Geometry check sheet. Reference: the model listing, model coordinates, mm. Face numbers are marked on the shaded views. A direction names the side the tool comes from. Coordinates: 2 decimals unless noted, no trailing zeros. Order: outer loops, then holes, each group sorted by start corner. A loop starts at its lowest first (then second) coordinate and runs counter-clockwise, first axis right, second up. Notation, with made-up numbers: (13.5, -12.5) -> (26.5, -12.5) arc R14 cw to (26.5, 1.5) -> close; hole circle Ø6 at (29, 72.5). An arc over 180 degrees is marked (long way). Answer in a Markdown table with one row per item. Add a question column.
```python
from build123d import *

# Parameters (mm, degrees)
EXTRUDE_1_DEPTH     = 100
FILLET_1_R          = 4
EXTRUDE_2_DEPTH     = 50
FILLET_2_R          = 1
CUT_EXTRUDE_1_DEPTH = 155.597772267
FILLET_3_R          = 1
CUT_EXTRUDE_2_REACH = 157.823
SKETCH_4_R          = 2.099999206


with BuildPart() as part:
    # 草图1 → 凸台-拉伸1 (new, symmetric)
    with BuildSketch(Plane.XY):
        Polygon((-30.1, 0), (30.1, 0), (0, 30.003999733), align=None)
    extrude(amount=EXTRUDE_1_DEPTH, both=True)

    # 圆角1
    fillet_1_edges = [part.edges().sort_by_distance(p)[0] for p in [
        (0, 30.003999733, 0),
        (30.1, 0, 0),
        (-30.1, 0, 0),
    ]]
    fillet(fillet_1_edges, radius=FILLET_1_R)

    # 草图2 → 凸台-拉伸2 (add)
    with BuildSketch(Plane.XY.offset(100)):
        Polygon((15.581935613, 6), (0, 21.532238936), (-15.581935613, 6), align=None)
    extrude(amount=EXTRUDE_2_DEPTH)

    # 圆角2
    fillet_2_edges = [part.edges().sort_by_distance(p)[0] for p in [
        (-15.581935613, 6, 125),
        (15.581935613, 6, 125),
        (0, 21.532238936, 125),
    ]]
    fillet(fillet_2_edges, radius=FILLET_2_R)

    # 草图3 → 切除-拉伸1 (cut, through all)
    with BuildSketch(Plane(origin=(0, 0, 0), x_dir=(1, 0, 0), z_dir=(0, 1, 0))):
        Polygon((-15, 82), (0, 67), (15, 82), align=None)
        Polygon((-8, 55), (-18, 35), (-2.823905857, 40), align=None)
        Polygon((2.823905857, 40), (8, 55), (18, 35), align=None)
        Polygon((8, 5), (18, 25), (2.823905857, 20), align=None)
        Polygon((-2.823905857, 20), (-8, 5), (-18, 25), align=None)
        Polygon((-8, -5), (-18, -25), (-2.823905857, -20), align=None)
        Polygon((2.823905857, -20), (8, -5), (18, -25), align=None)
        Polygon((8, -55), (18, -35), (2.823905857, -40), align=None)
        Polygon((-2.823905857, -40), (-8, -55), (-18, -35), align=None)
        Polygon((15, -82), (0, -67), (-15, -82), align=None)
    extrude(amount=CUT_EXTRUDE_1_DEPTH, mode=Mode.SUBTRACT)

    # 圆角3
    fillet_3_edges = [part.edges().sort_by_distance(p)[0] for p in [
        (0, 14.178079601, -67),
        (-15, 7.525920199, -82),
        (2.823905857, 13.594550189, -40),
        (8, 11.014757377, -55),
        (18, 6.030704265, -35),
        (-2.823905857, 13.594550189, -20),
        (-8, 11.014757377, -5),
        (-18, 6.030704265, -25),
        (2.823905857, 13.594550189, 20),
        (8, 11.014757377, 5),
        (18, 6.030704265, 25),
        (-2.823905857, 13.594550189, 40),
        (-8, 11.014757377, 55),
        (-18, 6.030704265, 35),
        (-15, 7.525920199, 82),
        (0, 14.178079601, 67),
        (15, 7.525920199, 82),
        (2.823905857, 13.594550189, 40),
        (18, 6.030704265, 35),
        (8, 11.014757377, 55),
        (-2.823905857, 13.594550189, 20),
        (-18, 6.030704265, 25),
        (-8, 11.014757377, 5),
        (2.823905857, 13.594550189, -20),
        (18, 6.030704265, -25),
        (8, 11.014757377, -5),
        (-2.823905857, 13.594550189, -40),
        (-18, 6.030704265, -35),
        (-8, 11.014757377, -55),
        (15, 7.525920199, -82),
    ]]
    fillet(fillet_3_edges, radius=FILLET_3_R)

    # 草图4 → 切除-拉伸2 (cut, up to next)
    with BuildSketch(Plane(origin=(-15.001923322, 15.04992321, 0), x_dir=(0.7082352941176472, 0.705976464314562, 0), z_dir=(-0.705976464314562, 0.7082352941176472, 0)), mode=Mode.PRIVATE) as cut_extrude_2_sk1:
        with Locations(Location((5.355142644, 85, 0), (0, 0, 180))):
            Circle(SKETCH_4_R)
    cut_extrude_2_tool1 = extrude(cut_extrude_2_sk1.sketch, amount=-CUT_EXTRUDE_2_REACH, mode=Mode.PRIVATE) & part.part
    cut_extrude_2 = cut_extrude_2_tool1.solids().sort_by_distance((-11.209222, 18.830528, -85))[0]
    add(cut_extrude_2, mode=Mode.SUBTRACT)

    # 镜向1: 切除-拉伸2 mirrored; each copy of 切除-拉伸2 runs up to whatever stops it at its own place
    mirror_1_before = part.part  # the part as the pattern finds it: every copy runs up to it
    mirror_1_cut_extrude_2_long = extrude(cut_extrude_2_sk1.sketch, amount=-CUT_EXTRUDE_2_REACH, mode=Mode.PRIVATE)
    mirror_1_cut_extrude_2_tool1 = mirror_1_cut_extrude_2_long.mirror(Plane(origin=(0, 0, 0), x_dir=(0, 0, 1), z_dir=(1, 0, 0))) & mirror_1_before
    add(mirror_1_cut_extrude_2_tool1.solids().sort_by_distance((11.209222, 18.830528, -85))[0], mode=Mode.SUBTRACT)


solid = part.part
```
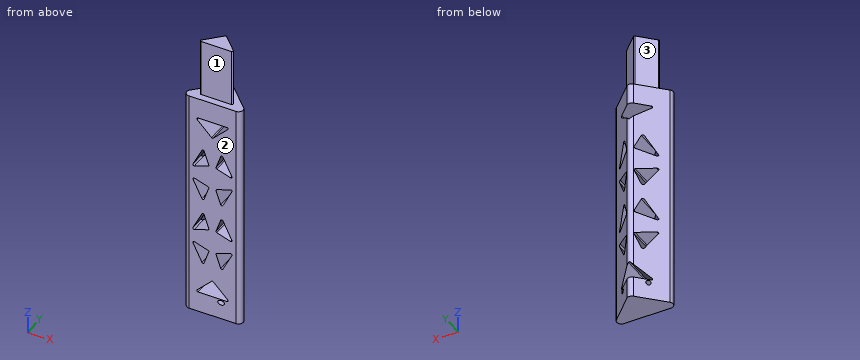
(1) Cross-section at B-B (y = 3). Give the number of separate pieces and of enclosed holes in the cut face, plus the area to 3 significant figures.
(2) Cross-section at C-C (z = 115). Enter the section's corners in (x, y).
(3) Cross-section at A-A (z = 27). Enter the section's corners in (x, y), plus the area to 3 significant figures.
(4) Access from +Z, -Z, +X, -X, +Y, -Y to the whole of each face (thin tool, end or side, straight path). Record for the marked faces 1, 2 and 3.
(5) Scan lines: line 1 along Z through (x, y) = (14, 10); line 2 along X through (y, z) = (10.25, -50.5); line 3 along X through (y, z) = (12.75, 16.5). Record each from-to range of solid material in increasing order.
(6) Go/stop test with flat-tipped pins: P1, Ø21, axis at x = 6, z = 118.5, coming from the -Y side; P2, Ø8, axis at x = 3.5, z = 46.5, coming from the +Y side; P3, Ø1, axis at y = 13, z = 94.5, coming from the +X side; P4, Ø10, axis at y = 24, z = -66.5, coming from the -X side. Record where each tip stops, or that it passes through.
Checks:
| question | item | result |
|---|---|---|
| 1 | separate pieces | 1 |
| 1 | enclosed holes | 11 |
| 1 | area | 8,260 mm² |
| 2 | outline | (-13.87, 7.71) arc R1 ccw to (-13.16, 6) -> (13.16, 6) arc R1 ccw to (13.87, 7.71) -> (0.71, 20.83) arc R1 ccw to (-0.71, 20.83) -> close |
| 3 | outline | (-23.25, 6.83) arc R4 ccw to (-20.42, 0) -> (20.42, 0) arc R4 ccw to (23.25, 6.83) -> (2.82, 27.19) arc R4 ccw to (-2.82, 27.19) -> close |
| 3 | area | 860 mm² |
| 4 | face 1 | +Z, +X, -X, -Y |
| 4 | face 2 | +Z, -Z, +X, -X, -Y |
| 4 | face 3 | +Z, -X, +Y |
| 5 | line 1 | -100 to -43, -36.32 to -23.68, -17 to 17, 23.68 to 36.32, 43 to 100 |
| 5 | line 2 | -19.82 to -10.25, -6.45 to 6.45, 10.25 to 19.82 |
| 5 | line 3 | -17.31 to -13.75, -4.03 to 4.03, 13.75 to 17.31 |
| 6 | P1 | y = 6 |
| 6 | P2 | y = 28.36 |
| 6 | P3 | x = 17.56 |
| 6 | P4 | x = -11.04 |
